Here's the drawing with two shaded views (mm, measured from the low corner). I have some questions. Give positions to 0.01 mm unless a question says otherwise; leave off trailing zeros. Write each loop counter-clockwise with the first axis right and the second up, starting at its lowest first coordinate (ties: lowest second). Pieces come first, ordered by that corner, then holes. Notation, with made-up numbers: (-10, 13.5) - (45, 13.5) arc R19 cw to (45, 33.5) - close; hole circle Ø7 at (6, -13.75). An arc over 180 degrees is marked (long way). Answer as a JSON object with one key per item and string values. Group by question number.
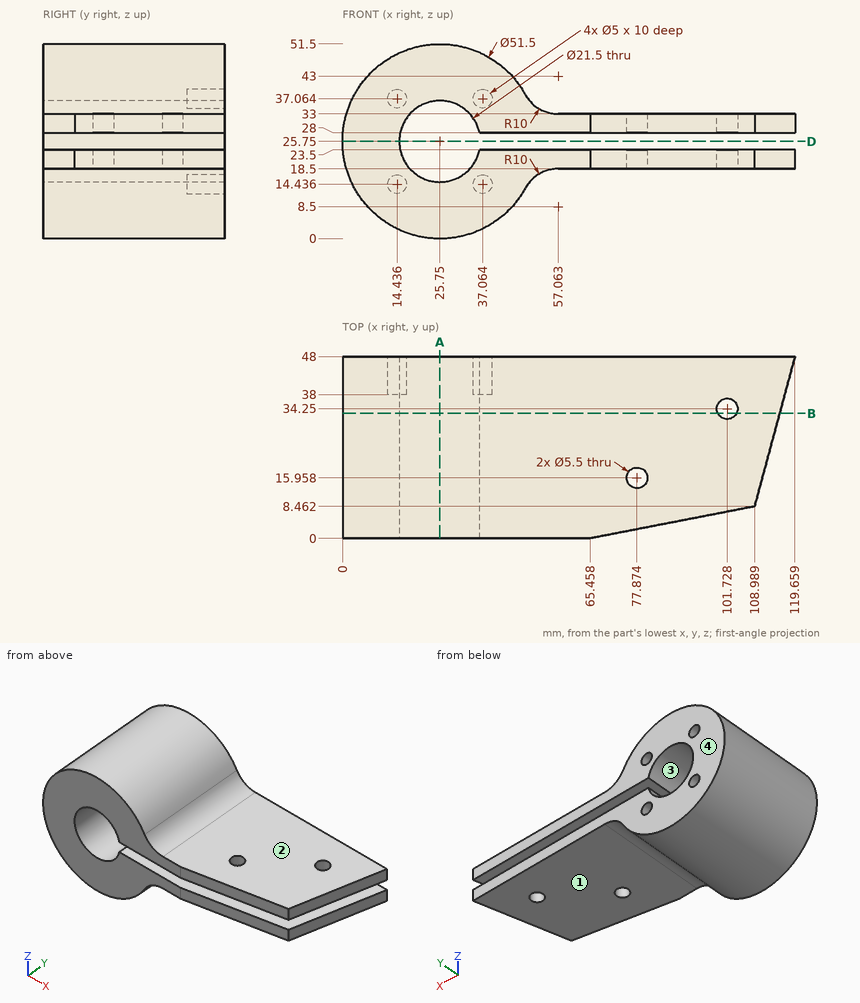
(1) Will these pins go through, and if not, where does the flat tip stop? P1, Ø1.5, axis at x = 71, y = 9.5, coming from the +Z side; P2, Ø4.5, axis at x = 37.06, z = 14.44, coming from the +Y side; P3, Ø2, axis at y = 10.5, z = 32.5, coming from the -X side; P4, Ø4.5, axis at x = 101.73, y = 34.25, coming from the -Z side.
(2) If we mould it in two halves opening along Z, with no side actions, what happens to the marked faces 1, 2, 3 and 4? For each: +Z half, -Z half, draft (parallel to the pull), parting line (faces both ways), or undercut.
(3) I need wall thicknesses on L1, parallel to Z at x = 81.5, y = 16; L2, parallel to Z at x = 37.5, y = 24; L3, parallel to X at y = 41.5, z = 23 (1 decimal). Which ranges of each line are inside material? Lowest first, please.
(4) I want a section at A-A, the plane x = 25.75. Please give me the cut outline in (y, z), and give its area (3 significant figures).
(5) I want a section at B-B, the plane y = 33. State how many separate pieces and enclosed holes the cut face has, and give its area (3 significant figures).
(6) I want a section at D-D, the plane z = 25.75. Please give me the cut outline in (x, y), and give its area (3 significant figures).
Entries:
{
 "1": {"P1": "z = 33", "P2": "y = 38", "P3": "x = 0.65", "P4": "through"},
 "2": {"face 1": "-Z half", "face 2": "+Z half", "face 3": "undercut", "face 4": "draft"},
 "3": {"L1": "18.5 to 23.5, 28 to 33", "L2": "2.84 to 23.5, 28 to 48.66", "L3": "0.1 to 15.4, 36.1 to 117.9"},
 "4": {"outline": "(0, 0) - (48, 0) - (48, 15) - (0, 15) - close; (0, 36.5) - (48, 36.5) - (48, 51.5) - (0, 51.5) - close", "area": "1,440 mm^2"},
 "5": {"separate pieces": "3", "enclosed holes": "0", "area": "2,260 mm^2"},
 "6": {"outline": "(0, 0) - (15, 0) - (15, 48) - (0, 48) - close", "area": "720 mm^2"}
}
